Design review of the part built by this model. Coordinates are the model's own, in mm. Round coordinates to 2 decimals unless told otherwise and drop trailing zeros. Write each loop counter-clockwise with the first axis right and the second up, starting at its lowest first coordinate (ties: lowest second). Pieces come first, ordered by that corner, then holes.
from build123d import *

# Parameters (mm, degrees)
F0_W     = 450
F0_H     = 450
F1_DEPTH = 18
F2_W     = 430
F2_H     = 5
F3_DEPTH = 8


with BuildPart() as f1:
    # F0 (on Front) → F1 (new body)
    with BuildSketch(Plane.XZ):
        Rectangle(F0_W, F0_H)
    extrude(amount=-F1_DEPTH)

    # F2 (on face) → F3 (cut)
    with BuildSketch(Plane.XZ):
        with Locations((10, 214.5)):
            Rectangle(F2_W, F2_H)
        with Locations((10, 204.5)):
            Rectangle(F2_W, F2_H)
        with Locations((10, 194.5)):
            Rectangle(F2_W, F2_H)
        with Locations((10, 184.5)):
            Rectangle(F2_W, F2_H)
    extrude(amount=-F3_DEPTH, mode=Mode.SUBTRACT)


solid = f1.part
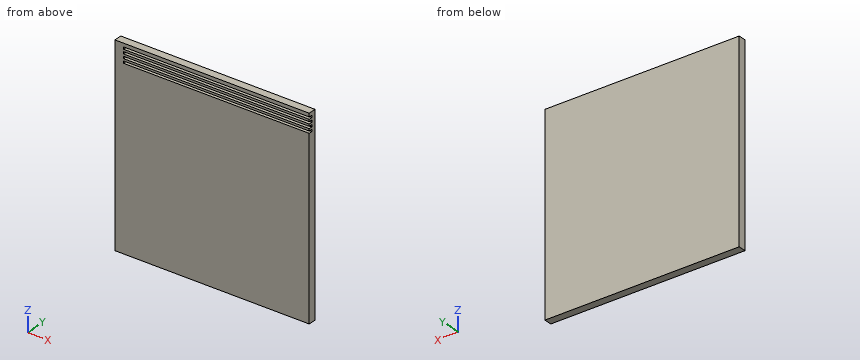
1) Add section A-A on x = 1. State the section outline as (y, z) points, and give its area (3 significant figures).
2) For P1, Ø2.5, axis at x = -2.5, z = 193.5, coming from the -Y side; P2, Ø2.5, axis at y = 2.5, z = 214, coming from the +X side; P3, Ø4, axis at x = 2.5, z = 215.5, coming from the -Y side, all flat-tipped, find the tip position at first contact; note any pin that passes through.
3) Add section B-B on y = 5. State the section outline as (x, z) points.
4) For line 1 along Z through (x, y) = (-101.5, 3.75), list the stretches that pass through material, from the lowest coordinate up.
Computed:
1. outline: (0, -225) - (18, -225) - (18, 225) - (0, 225) - (0, 217) - (8, 217) - (8, 212) - (0, 212) - (0, 207) - (8, 207) - (8, 202) - (0, 202) - (0, 197) - (8, 197) - (8, 192) - (0, 192) - (0, 187) - (8, 187) - (8, 182) - (0, 182) - close
1. area: 7,940 mm2
2. P1: stops at y = 8
2. P2: stops at x = -205
2. P3: stops at y = 0
3. outline: (-225, -225) - (225, -225) - (225, 182) - (-205, 182) - (-205, 187) - (225, 187) - (225, 192) - (-205, 192) - (-205, 197) - (225, 197) - (225, 202) - (-205, 202) - (-205, 207) - (225, 207) - (225, 212) - (-205, 212) - (-205, 217) - (225, 217) - (225, 225) - (-225, 225) - close
4. line 1: z = -225 to 182, 187 to 192, 197 to 202, 207 to 212, 217 to 225
